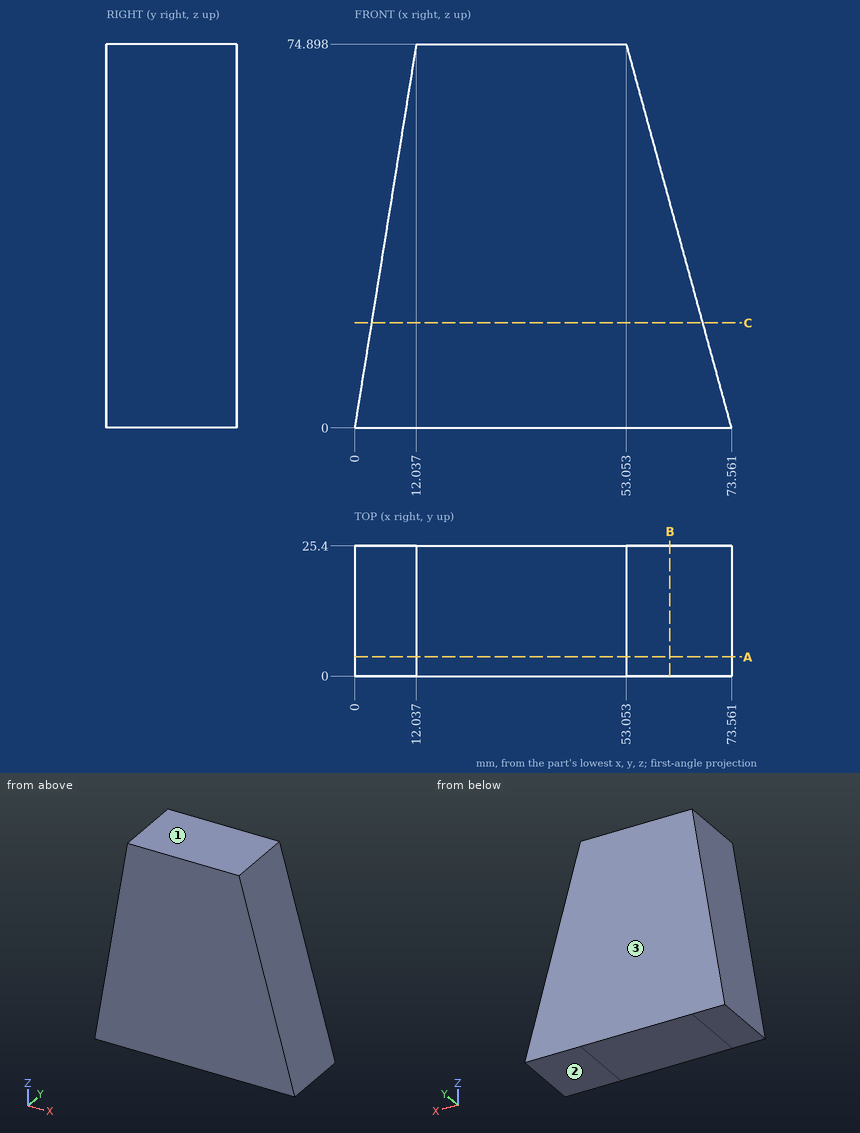
Part print with two shaded views. Sizes in mm from the minimum x, y, z corner. Coordinates: 2 decimals unless noted, no trailing zeros. Order: outer loops, then holes, each group sorted by start corner. A loop starts at its lowest first (then second) coordinate and runs counter-clockwise, first axis right, second up. Notation, with made-up numbers: (10, 14.25) - (59, 14.25) arc R18 ccw to (59, 26.25) - close; hole circle Ø9 at (5.5, 59). An arc over 180 degrees is marked (long way). Write item = value, one per line. Start each with the question number.
1) Saw through at A-A on y = 3.75. Write the cut outline in (x, z).
2) Two-plate mould, pull along Z, no slides. Class the marked faces 1, 2 and 3: pulls with the +Z half, pulls with the -Z half, needs draft (parallel to the pull), parting line crosses it, or undercut.
3) Flat gauge pins, fed straight in: pin 1 Ø10 at (y, z) = (7, 62.5) entering from +X; pin 2 Ø2 at (y, z) = (17, 31.5) entering from -X; pin 3 Ø5 at (y, z) = (3.5, 37.5) entering from -X (1 decimal). Where does each tip first touch, or does it go through?
4) Wall check: line 1 along X through (y, z) = (17, 21.5) (1 decimal); line 2 along X through (y, z) = (4, 28) (1 decimal). Give the ranges that are in metal, low to high. Write a range as from..to.
5) Saw through at B-B on x = 61.5. Write the cut outline in (y, z), then the cut area to 3 significant figures.
6) Saw through at C-C on z = 20.5. Write the cut outline in (x, y) (1 decimal).
From the geometry:
q1.outline = (0, 0) - (73.56, 0) - (53.05, 74.9) - (12.04, 74.9) - close
q2.face_1 = pulls with the +Z half
q2.face_2 = pulls with the -Z half
q2.face_3 = needs draft
q3.pin_1 = 57.82
q3.pin_2 = 4.9
q3.pin_3 = 5.6
q4.line_1 = 3.5..67.7
q4.line_2 = 4.5..65.9
q5.outline = (0, 0) - (25.4, 0) - (25.4, 44.05) - (0, 44.05) - close
q5.area = 1,120 mm^2
q6.outline = (3.3, 0) - (67.9, 0) - (67.9, 25.4) - (3.3, 25.4) - close
